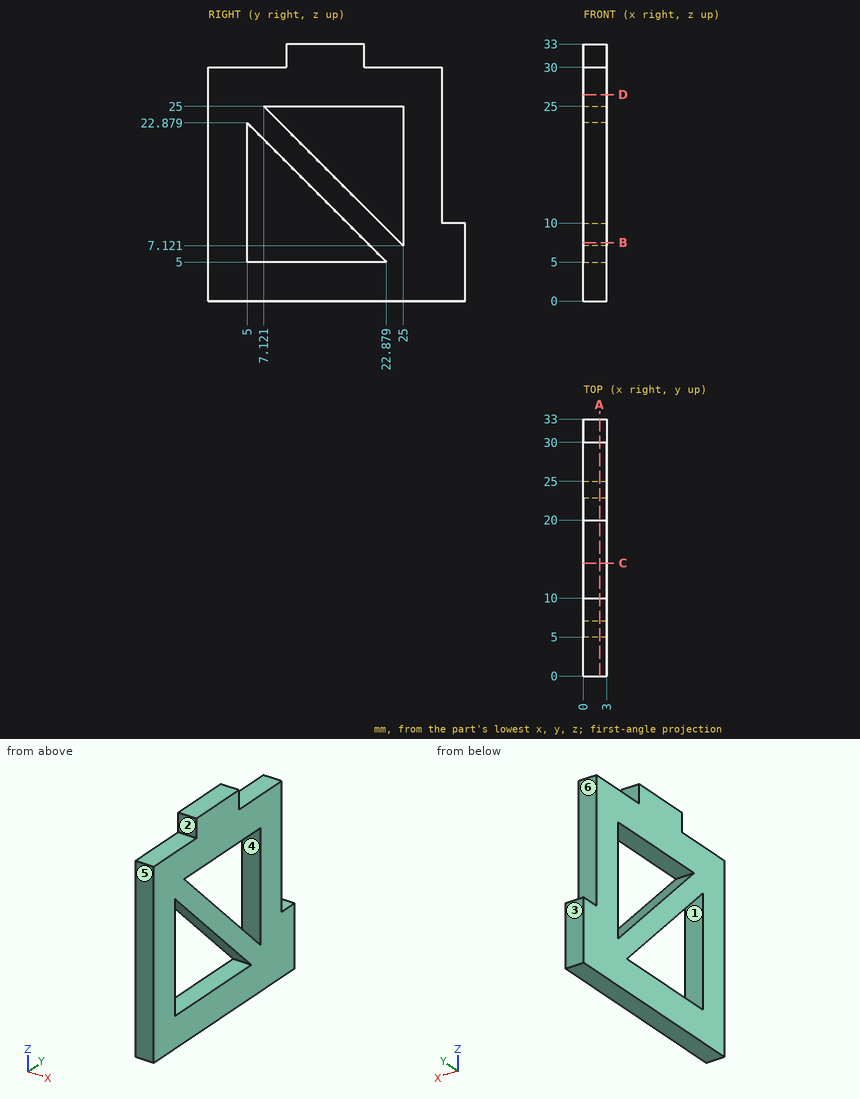
Part print with two shaded views. Sizes in mm from the minimum x, y, z corner. A direction names the side the tool comes from. Round coordinates to 2 decimals unless told otherwise and drop trailing zeros. Order: outer loops, then holes, each group sorted by start corner. A loop starts at its lowest first (then second) coordinate and runs counter-clockwise, first axis right, second up.
(1) Drill centre lines: line 1 (Y direction, x = 1.7, z = 12.5); line 2 (Z direction, x = 1.3, y = 18); line 3 (Y direction, x = 1.4, z = 19). Where is each one in solid material? Low to high.
(2) Band-saw the part on B-B (z = 7.5). List the corners of the cut face in (x, y).
(3) 3-axis set-ups, long thin cutter, end or side, ignore diameter. For the marked faces 1, 2 and 3: which of +Z, -Z, +X, -X, +Y, -Y reach the whole face in a straight line?
(4) Band-saw the part on C-C (y = 14.5). List the corners of the cut face in (x, z).
(5) Band-saw the part on A-A (x = 2.1). List the corners of the cut face in (y, z).
(6) Band-saw the part on D-D (z = 26.5). List the corners of the cut face in (x, y).
(7) Pin check, flat tips, straight feed: pin 1 (1.5 mm diameter, centred on x = 1.5, z = 23, fed in from +Y); pin 2 (0.9 mm diameter, centred on x = 1.5, z = 13, fed in from -Y); pin 3 (0.9 mm diameter, centred on x = 1.5, y = 5, fed in from +Z); pin 4 (1.5 mm diameter, centred on x = 2, z = 31.5, fed in from +Y). Stop position of each tip, or through.
(8) Pull direction Y, two halves, no side cores. Call the marked faces 4, 5 and 6: released by +Y, released by -Y, zero draft, split by the parting line, or undercut.
Verdict:
1. line 1: y = 0 to 5, 15.38 to 19.62, 25 to 30
1. line 2: z = 0 to 5, 9.88 to 14.12, 25 to 33
1. line 3: y = 0 to 5, 8.88 to 13.12, 25 to 30
2. outline: (0, 0) - (3, 0) - (3, 5) - (0, 5) - close; (0, 20.38) - (3, 20.38) - (3, 24.62) - (0, 24.62) - close; (0, 25) - (3, 25) - (3, 33) - (0, 33) - close
3. face 1: +X, -X
3. face 2: +Z, +X, -X, -Y
3. face 3: +Z, -Z, +X, -X, +Y
4. outline: (0, 0) - (3, 0) - (3, 5) - (0, 5) - close; (0, 13.38) - (3, 13.38) - (3, 17.62) - (0, 17.62) - close; (0, 25) - (3, 25) - (3, 33) - (0, 33) - close
5. outline: (0, 0) - (33, 0) - (33, 10) - (30, 10) - (30, 30) - (20, 30) - (20, 33) - (10, 33) - (10, 30) - (0, 30) - close; hole (5, 5) - (22.88, 5) - (5, 22.88) - close; hole (7.12, 25) - (25, 7.12) - (25, 25) - close
6. outline: (0, 0) - (3, 0) - (3, 30) - (0, 30) - close
7. pin 1: stops at y = 30
7. pin 2: stops at y = 0
7. pin 3: stops at z = 30
7. pin 4: stops at y = 20
8. face 4: undercut
8. face 5: released by -Y
8. face 6: released by +Y
